from build123d import *

# Parameters (mm, degrees)
SKETCH2_R                    = 3.15
BASE_FLANGE1_DEPTH           = 3.175
EDGE_FLANGE1_STRIP_W         = 19.05
EDGE_FLANGE1_STRIP_H         = 3.175
EDGE_FLANGE1_STRIP_CUT_DEPTH = 37
EDGE_FLANGE1_DEPTH           = 37
SKETCH10_R                   = 3.15
CUT_EXTRUDE1_DEPTH           = 10


# Sheet-metal steps are written as plain solids
with BuildPart() as part:
    # Sketch2 → Base-Flange1 (new body)
    with BuildSketch(Plane(origin=(0, 0, 0), x_dir=(0, 0, -1), z_dir=(1, 0, 0))):
        with BuildLine():
            Line((48.551064785, 40.291218586), (48.551064785, 72.093066751))
            Line((48.551064785, 72.093066751), (14.602650648, 58.297559694))
            ThreePointArc((14.602650648, 58.297559694), (12.37556545, 56.443388888), (11.551064785, 53.665249851))
            Line((11.551064785, 53.665249851), (11.551064785, 40.291218586))
            Line((11.551064785, 40.291218586), (48.551064785, 40.291218586))
        make_face()
        with Locations((39.011220588, 57.194773579)):
            Circle(SKETCH2_R, mode=Mode.SUBTRACT)
        with Locations((20.490203266, 52.672523101)):
            Circle(SKETCH2_R, mode=Mode.SUBTRACT)
    extrude(amount=-BASE_FLANGE1_DEPTH)

    # Edge-Flange1 strip (across the edge) → Edge-Flange1 strip cut (cut)
    with BuildSketch(Plane(origin=(0, 40.291218586, -11.551064785), x_dir=(0, 1, 0), z_dir=(0, 0, -1))):
        with Locations((-3.175, -1.5875)):
            Rectangle(EDGE_FLANGE1_STRIP_W, EDGE_FLANGE1_STRIP_H)
    extrude(amount=EDGE_FLANGE1_STRIP_CUT_DEPTH, mode=Mode.SUBTRACT)

    # Edge-Flange1 section (across the edge) → Edge-Flange1 (add)
    with BuildSketch(Plane(origin=(0, 40.291218586, -11.551064785), x_dir=(0, 1, 0), z_dir=(0, 0, -1))):
        with BuildLine():
            Line((0, 3.175), (0, 12.825))
            Line((0, 12.825), (3.175, 12.825))
            Line((3.175, 12.825), (3.175, 3.175))
            ThreePointArc((3.175, 3.175), (4.10493597, 0.92993597), (6.35, 0))
            Line((6.35, 0), (6.35, -3.175))
            ThreePointArc((6.35, -3.175), (1.859871939, -1.315128061), (0, 3.175))
        make_face()
    extrude(amount=EDGE_FLANGE1_DEPTH)

    # Sketch10 → Cut-Extrude1 (cut)
    with BuildSketch(Plane(origin=(0, 43.466218586, 0), x_dir=(1, 0, 0), z_dir=(0, 1, 0))):
        with Locations(Location((8, 40.102300831, 0), (0, 0, 180))):
            Circle(SKETCH10_R)
        with Locations(Location((8, 20.102300831, 0), (0, 0, 180))):
            Circle(SKETCH10_R)
    extrude(amount=-CUT_EXTRUDE1_DEPTH, mode=Mode.SUBTRACT)


solid = part.part
Build history of the part. All positions in model axes, mm. A direction names the side the tool comes from. Give positions to 0.01 mm unless a question says otherwise; leave off trailing zeros. Order: outer loops, then holes, each group sorted by start corner. A loop starts at its lowest first (then second) coordinate and runs counter-clockwise, first axis right, second up. Notation, with made-up numbers: M -30.5,-39.5 L 11.5,-39.5 A8 cw 11.5,-34.5 Z; hole C -29,42 d9. An arc over 180 degrees is marked long. Use one line per item in the form item = value.
1) Saw through at B-B (z = -21). Give the cut face in (x, y) (3 decimals).
Calculated:
outline = M -3.175,46.641 A6.35 ccw 3.175,40.291 L 4.981,40.291 L 4.981,43.466 L 3.175,43.466 A3.175 cw 0,46.641 L 0,49.564 L -3.175,49.564 Z; M -3.175,55.781 L 0,55.781 L 0,60.897 L -3.175,60.897 Z; M 11.019,40.291 L 12.825,40.291 L 12.825,43.466 L 11.019,43.466 Z
2) Probe probe 1 along Z at (x, y) = (8, 42.2); probe 2 along X at (y, z) = (63, -32.5) (3 decimals); probe 3 along Y at (x, z) = (-0.25, -38.5). List the from-to ranges inside material, lowest first.
Calculated:
probe_1 = -48.55 to -43.25, -36.95 to -23.25, -16.95 to -11.55
probe_2 = -3.175 to 0
probe_3 = 41.29 to 54.09, 60.3 to 68.01
3) Saw through at C-C (x = -0.75). Give the cut face in (y, z).
Calculated:
outline = M 41.65,-48.55 L 72.09,-48.55 L 58.3,-14.6 A5 ccw 53.67,-11.55 L 41.65,-11.55 Z; hole C 52.67,-20.49 d6.3; hole C 57.19,-39.01 d6.3
4) Saw through at A-A (x = 8). Give the cut face in (y, z), plus the area to 3 significant figures.
Calculated:
outline = M 40.29,-48.55 L 43.47,-48.55 L 43.47,-43.25 L 40.29,-43.25 Z; M 40.29,-36.95 L 43.47,-36.95 L 43.47,-23.25 L 40.29,-23.25 Z; M 40.29,-16.95 L 43.47,-16.95 L 43.47,-11.55 L 40.29,-11.55 Z
area = 77.5 mm2
5) Tool access for faces 4 (the face through (8, 43.466, -30)), 5 (the face through (-1.565, 54.4, -40.465)): list every direction of +Z, -Z, +X, -X, +Y, -Y with a clear straight run to the whole face (end or side of a thin tool).
Calculated:
face_4 = +Z, -Z, +X, +Y
face_5 = +X, -X
6) Two-plate mould, pull along Z, no slides. Class faces 1 (the face through (12.825, 42, -30)), 2 (the face through (2, 43, -11.551)), 3 (the face through (8.41, 41.9, -36.98)): released by +Z, released by -Z, zero draft, split by the parting line, or undercut.
Calculated:
face_1 = zero draft
face_2 = released by +Z
face_3 = undercut
7) Saw through at D-D (z = -31). Give the cut face in (x, y) (3 decimals).
Calculated:
outline = M -3.175,46.641 A6.35 ccw 3.175,40.291 L 12.825,40.291 L 12.825,43.466 L 3.175,43.466 A3.175 cw 0,46.641 L 0,64.961 L -3.175,64.961 Z
8) Drop flat-ended pins along their axis: pin 1 (1 mm diameter, centred on x = 3, z = -27.5, fed in from -Y); pin 2 (8 mm diameter, centred on x = 1, z = -25, fed in from +Y); pin 3 (4 mm diameter, centred on x = 7.5, z = -17, fed in from +Y); pin 4 (7.5 mm diameter, centred on y = 54.5, z = -25, fed in from +X). Give the stop position or say it passes through.
Calculated:
pin_1 = 40.29
pin_2 = 64.1
pin_3 = 43.47
pin_4 = 0
